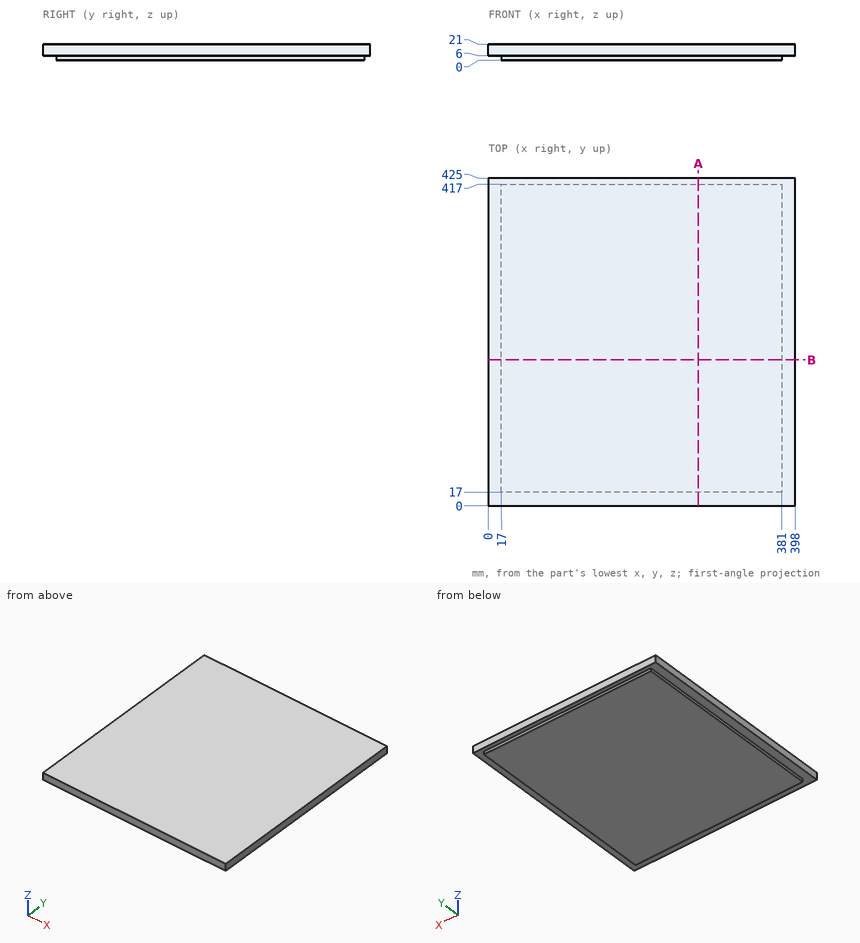
Verification items for this drawing (mm, ordinates from the low corner). Coordinates: 2 decimals unless noted, no trailing zeros. Order: outer loops, then holes, each group sorted by start corner. A loop starts at its lowest first (then second) coordinate and runs counter-clockwise, first axis right, second up. Notation, with made-up numbers: M 10,59.5 L 45,59.5 A21 cw 45,71.5 Z; hole C 41,27.5 d10. An arc over 180 degrees is marked long. Answer as a JSON object with one key per item and string values.
Q1. Cross-section at A-A on x = 272.5. Record the cut outline in (y, z).
Results are:
{"outline": "M 0,6 L 17,6 L 17,0 L 417,0 L 417,6 L 425,6 L 425,21 L 0,21 Z"}
Q2. Cross-section at B-B on y = 189. Record the cut outline in (x, z).
Results are:
{"outline": "M 0,6 L 17,6 L 17,0 L 381,0 L 381,6 L 398,6 L 398,21 L 0,21 Z"}
Q3. Scan lines: line 1 (Y direction, x = 269, z = 5); line 2 (X direction, y = 346, z = 2.25). Record each from-to range of solid material in increasing order.
Results are:
{"line 1": "y = 17 to 417", "line 2": "x = 17 to 381"}
Q4. Depth check by flat-ended pin: pin 1 Ø5 at (x, y) = (248, 105) entering from -Z; pin 2 Ø5 at (x, z) = (171, 1.5) entering from +Y; pin 3 Ø1.8 at (x, z) = (136.5, 4) entering from -Y; pin 4 Ø6.5 at (y, z) = (211.5, 2) entering from -X. Enter the tip coordinate at first touch or a pass-through.
Results are:
{"pin 1": "stops at z = 0", "pin 2": "stops at y = 417", "pin 3": "stops at y = 17", "pin 4": "stops at x = 17"}
